Here's how the part is built. I have some questions about the finished solid (model axes, mm). A direction names the side the tool comes from. Give positions to 0.01 mm unless a question says otherwise; leave off trailing zeros. Loops run counter-clockwise (first coordinate to the right, second up) from the corner with the lowest first, then second, coordinate; pieces in that order, holes last.
Q1. If we section it at D-D (y = -5): Please give me the cut outline in (x, z), plus the area to 3 significant figures.
Q2. Will these pins go through, and if not, where does the flat tip stop? P1, Ø4, axis at x = -2.5, z = 3.5, coming from the -Y side; P2, Ø3, axis at x = -0.5, y = 1, coming from the +Z side; P3, Ø4.5, axis at y = 3, z = 3, coming from the -X side.
Q3. We'd pull the mould along X, two halves only. Please class faces 4 (the face through (-1.46, -6.59, 3.94)), 5 (the face through (2.209, -5.037, 6.479)), 6 (the face through (0, 0, 0)): +X half, -X half, draft (parallel to the pull), parting line (faces both ways), or undercut.
Q4. I need wall thicknesses on line 1 (Y direction, x = 4.75, z = 2.5); line 2 (X direction, y = 4.5, z = 0.5); line 3 (X direction, y = 4.25, z = 1.5). Which ranges of each line are inside material? Lowest first, please.
Q5. If we section it at B-B (z = 1): Please give me the cut outline in (x, y), plus the area to 3 significant figures.
Q6. For faces 1 (the face through (1.47, 3.15, 2.46)), 2 (the face through (5.43, 0.87, 6.48)), 3 (the face through (-6, 0, 8)), which set-ups out of +Z, -Z, +X, -X, +Y, -Y let a thin tool reach every point of the face, with its end or its side?
Q7. If we section it at C-C (x = -0.5): Please give me the cut outline in (y, z), plus the area to 3 significant figures.
Q8. If we section it at A-A (y = 4.5): Please give me the cut outline in (x, z).
from build123d import *

# Parameters (mm, degrees)
F0_R     = 6.75
F1_DEPTH = 8
F2_DEPTH = 5


with BuildPart() as f1:
    # F0 (on Top) → F1 (new body)
    with BuildSketch(Plane.XY):
        Circle(F0_R)
        with BuildLine():
            ThreePointArc((5.230811, 1.699593), (5.432286, 0.86039), (5.5, 0))
            ThreePointArc((5.5, 0), (5.489741, -0.335767), (5.459004, -0.670281))
            ThreePointArc((5.459004, -0.670281), (4.73896, -2.791461), (3.232819, -4.449593))
            ThreePointArc((3.232819, -4.449593), (2.19312, -5.04383), (1.049449, -5.39895))
            ThreePointArc((1.049449, -5.39895), (-1.190418, -5.369628), (-3.232819, -4.449593))
            ThreePointArc((-3.232819, -4.449593), (-4.119256, -3.64441), (-4.810408, -2.666453))
            ThreePointArc((-4.810408, -2.666453), (-5.474679, -0.527152), (-5.230811, 1.699593))
            ThreePointArc((-5.230811, 1.699593), (-4.73896, 2.791461), (-4.022445, 3.750991))
            ThreePointArc((-4.022445, 3.750991), (-2.19312, 5.04383), (0, 5.5))
            ThreePointArc((0, 5.5), (1.190418, 5.369628), (2.3244, 4.984693))
            ThreePointArc((2.3244, 4.984693), (4.119256, 3.64441), (5.230811, 1.699593))
        make_face(mode=Mode.SUBTRACT)
    extrude(amount=F1_DEPTH)

    # F0 (on Top) → F2 (join)
    with BuildSketch(Plane.XY):
        Circle(F0_R)
        with BuildLine():
            ThreePointArc((5.230811, 1.699593), (5.432286, 0.86039), (5.5, 0))
            ThreePointArc((5.5, 0), (5.489741, -0.335767), (5.459004, -0.670281))
            ThreePointArc((5.459004, -0.670281), (4.73896, -2.791461), (3.232819, -4.449593))
            ThreePointArc((3.232819, -4.449593), (2.19312, -5.04383), (1.049449, -5.39895))
            ThreePointArc((1.049449, -5.39895), (-1.190418, -5.369628), (-3.232819, -4.449593))
            ThreePointArc((-3.232819, -4.449593), (-4.119256, -3.64441), (-4.810408, -2.666453))
            ThreePointArc((-4.810408, -2.666453), (-5.474679, -0.527152), (-5.230811, 1.699593))
            ThreePointArc((-5.230811, 1.699593), (-4.73896, 2.791461), (-4.022445, 3.750991))
            ThreePointArc((-4.022445, 3.750991), (-2.19312, 5.04383), (0, 5.5))
            ThreePointArc((0, 5.5), (1.190418, 5.369628), (2.3244, 4.984693))
            ThreePointArc((2.3244, 4.984693), (4.119256, 3.64441), (5.230811, 1.699593))
        make_face(mode=Mode.SUBTRACT)
        with BuildLine():
            Line((0.633927, 1.359462), (2.3244, 4.984693))
            ThreePointArc((2.3244, 4.984693), (1.190418, 5.369628), (0, 5.5))
            Line((0, 5.5), (0, 1.5))
            ThreePointArc((0, 1.5), (0.324659, 1.464444), (0.633927, 1.359462))
        make_face()
        with BuildLine():
            Line((-1.097031, 1.022998), (-4.022445, 3.750991))
            ThreePointArc((-4.022445, 3.750991), (-4.73896, 2.791461), (-5.230811, 1.699593))
            Line((-5.230811, 1.699593), (-1.426585, 0.463525))
            ThreePointArc((-1.426585, 0.463525), (-1.292444, 0.761308), (-1.097031, 1.022998))
        make_face()
        with BuildLine():
            ThreePointArc((-4.810408, -2.666453), (-4.119256, -3.64441), (-3.232819, -4.449593))
            Line((-3.232819, -4.449593), (-0.881678, -1.213525))
            ThreePointArc((-0.881678, -1.213525), (-1.123434, -0.99393), (-1.31193, -0.727214))
            Line((-1.31193, -0.727214), (-4.810408, -2.666453))
        make_face()
        with BuildLine():
            ThreePointArc((1.049449, -5.39895), (2.19312, -5.04383), (3.232819, -4.449593))
            Line((3.232819, -4.449593), (0.881678, -1.213525))
            ThreePointArc((0.881678, -1.213525), (0.598124, -1.37559), (0.286213, -1.472441))
            Line((0.286213, -1.472441), (1.049449, -5.39895))
        make_face()
        with BuildLine():
            ThreePointArc((5.459004, -0.670281), (5.489741, -0.335767), (5.5, 0))
            ThreePointArc((5.5, 0), (5.432286, 0.86039), (5.230811, 1.699593))
            Line((5.230811, 1.699593), (1.426585, 0.463525))
            ThreePointArc((1.426585, 0.463525), (1.481533, 0.234652), (1.5, 0))
            ThreePointArc((1.5, 0), (1.497202, -0.091573), (1.488819, -0.182804))
            Line((1.488819, -0.182804), (5.459004, -0.670281))
        make_face()
        with BuildLine():
            ThreePointArc((1.5, 0), (1.481533, 0.234652), (1.426585, 0.463525))
            ThreePointArc((1.426585, 0.463525), (1.123434, 0.99393), (0.633927, 1.359462))
            ThreePointArc((0.633927, 1.359462), (0.324659, 1.464444), (0, 1.5))
            ThreePointArc((0, 1.5), (-0.598124, 1.37559), (-1.097031, 1.022998))
            ThreePointArc((-1.097031, 1.022998), (-1.292444, 0.761308), (-1.426585, 0.463525))
            ThreePointArc((-1.426585, 0.463525), (-1.493094, -0.143769), (-1.31193, -0.727214))
            ThreePointArc((-1.31193, -0.727214), (-1.123434, -0.99393), (-0.881678, -1.213525))
            ThreePointArc((-0.881678, -1.213525), (-0.324659, -1.464444), (0.286213, -1.472441))
            ThreePointArc((0.286213, -1.472441), (0.598124, -1.37559), (0.881678, -1.213525))
            ThreePointArc((0.881678, -1.213525), (1.292444, -0.761308), (1.488819, -0.182804))
            ThreePointArc((1.488819, -0.182804), (1.497202, -0.091573), (1.5, 0))
        make_face()
    extrude(amount=F2_DEPTH)


solid = f1.part
Check sheet entries:
1. outline: (-4.53, 0) - (-2.29, 0) - (-2.29, 8) - (-4.53, 8) - close; (0.97, 0) - (4.53, 0) - (4.53, 8) - (2.29, 8) - (2.29, 5) - (0.97, 5) - close
1. area: 42.5 mm2
2. P1: stops at y = -6.73
2. P2: stops at z = 5
2. P3: stops at x = -6.71
3. face 4: parting line
3. face 5: undercut
3. face 6: draft
4. line 1: y = -4.8 to -2.77, -0.58 to 1.54, 2.77 to 4.8
4. line 2: x = -5.03 to -3.16, 0 to 2.1, 3.16 to 5.03
4. line 3: x = -5.24 to -3.49, 0 to 1.98, 3.49 to 5.24
5. outline: circle Ø13.5 at (0, 0); hole (-5.23, 1.7) arc R5.5 ccw to (-4.81, -2.67) - (-1.31, -0.73) arc R1.5 cw to (-1.43, 0.46) - close; hole (-4.02, 3.75) - (-1.1, 1.02) arc R1.5 cw to (0, 1.5) - (0, 5.5) arc R5.5 ccw to start; hole (-3.23, -4.45) arc R5.5 ccw to (1.05, -5.4) - (0.29, -1.47) arc R1.5 cw to (-0.88, -1.21) - close; hole (0.63, 1.36) arc R1.5 cw to (1.43, 0.46) - (5.23, 1.7) arc R5.5 ccw to (2.32, 4.98) - close; hole (0.88, -1.21) - (3.23, -4.45) arc R5.5 ccw to (5.46, -0.67) - (1.49, -0.18) arc R1.5 cw to start
5. area: 85.7 mm2
6. face 1: +Z, -Z
6. face 2: +Z
6. face 3: +Z, +X, -X, +Y, -Y
7. outline: (-6.73, 0) - (-5.48, 0) - (-5.48, 8) - (-6.73, 8) - close; (-1.41, 0) - (1.41, 0) - (1.41, 5) - (-1.41, 5) - close; (5.48, 0) - (6.73, 0) - (6.73, 8) - (5.48, 8) - close
7. area: 34.2 mm2
8. outline: (-5.03, 0) - (-3.16, 0) - (-3.16, 8) - (-5.03, 8) - close; (0, 0) - (2.1, 0) - (2.1, 5) - (0, 5) - close; (3.16, 0) - (5.03, 0) - (5.03, 8) - (3.16, 8) - close
